from build123d import *

# Parameters (mm, degrees)
F1_DEPTH = 29
F2_R     = 10
F3_DEPTH = 20.001
F4_W     = 9.6138500422
F4_H     = 3
F5_DEPTH = 20.001
F7_D     = 6.3


with BuildPart() as f1:
    # F0 (on Top) → F1 (new body)
    with BuildSketch(Plane.XY):
        Polygon((20, 5), (15, 10), (-15, 10), (-20, 5), (-20, -5), (-15, -10), (15, -10), (20, -5), align=None)
    extrude(amount=F1_DEPTH)

    # F2 (on face) → F3 (cut, through all)
    with BuildSketch(Plane.XZ.offset(10)):
        with Locations((0, 13)):
            Circle(F2_R)
    extrude(amount=-F3_DEPTH, mode=Mode.SUBTRACT)

    # F4 (on face) → F5 (cut, through all)
    with BuildSketch(Plane.XZ.offset(10)):
        with Locations((-19.8069250211, 13)):
            Rectangle(F4_W, F4_H)
        with BuildLine():
            Line((-9.8868599666, 11.5), (-4.6138500422, 11.5))
            Line((-4.6138500422, 11.5), (-4.6138500422, 14.5))
            Line((-4.6138500422, 14.5), (-9.8868599666, 14.5))
            ThreePointArc((-9.8868599666, 14.5), (-10, 13), (-9.8868599666, 11.5))
        make_face()
        with BuildLine():
            Line((-15, 11.5), (-9.8868599666, 11.5))
            ThreePointArc((-9.8868599666, 11.5), (-10, 13), (-9.8868599666, 14.5))
            Line((-9.8868599666, 14.5), (-15, 14.5))
            Line((-15, 14.5), (-15, 11.5))
        make_face()
    extrude(amount=-F5_DEPTH, mode=Mode.SUBTRACT)

    # F7 (through all)
    with Locations(Plane.XY.offset(29)):
        with Locations((-15, 0), (15, 0)):
            Hole(F7_D / 2)


solid = f1.part
The listing builds one solid part. Answer for the finished solid, in the listing's coordinates (mm). A direction names the side the tool comes from. Round coordinates to 2 decimals unless told otherwise and drop trailing zeros. Write each loop counter-clockwise with the first axis right and the second up, starting at its lowest first coordinate (ties: lowest second). Pieces come first, ordered by that corner, then holes. Notation, with made-up numbers: (47.5, 10.25) - (62.5, 10.25) arc R35 cw to (62.5, 43.25) - close; hole circle Ø7 at (42, 5). An arc over 180 degrees is marked (long way). Use a Markdown table: item, result. Add a question column.
1. A flat-ended cylindrical pin translates along its axis: P1, Ø1, axis at x = 12.5, y = 4.5, coming from the -Z side. Find the tip coordinate at first contact, or state that the pin passes through.
2. The part is cut by section C-C (x = 0). Write down the section's boundary in (y, z).
3. The part is cut by section A-A (y = 0). Write down the section's boundary in (x, z).
4. A tool of negligible diameter and unlimited length cuts with its end or side. For faces 4 (the face through (-11.5, -0.1, 14.5)), 5 (the face through (-7, -10, 21)), from which of +Z, -Z, +X, -X, +Y, -Y can it reach the whole face along a straight path? Write none if from no direction.
5. Consider line 1 (Z direction, x = -17.5, y = -6.25); line 2 (Y direction, x = -15, z = 3.5); line 3 (X direction, y = 2.5, z = 20.5). Determine where each line is inside the solid, lowest interval first.
6. For a pull along Y with two mould halves and no side action, classify faces 1 (the face through (18.147, 0.138, 14.297)), 2 (the face through (-17, 8, 6)), 3 (the face through (-11.6, -0.1, 11.5)) as +Y half, -Y half, draft (parallel to the pull), parting line (faces both ways), or undercut.
7. The part is cut by section D-D (z = 17.25). Write down the section's boundary in (x, y), and give its area (3 significant figures).
8. The part is cut by section B-B (z = 13). Write down the section's boundary in (x, y), and give its area (3 significant figures).
Reported:
| question | item | result |
|---|---|---|
| 1 | P1 | z = 0 |
| 2 | outline | (-10, 0) - (10, 0) - (10, 3) - (-10, 3) - close; (-10, 23) - (10, 23) - (10, 29) - (-10, 29) - close |
| 3 | outline | (-20, 0) - (-18.15, 0) - (-18.15, 11.5) - (-20, 11.5) - close; (-20, 14.5) - (-18.15, 14.5) - (-18.15, 29) - (-20, 29) - close; (-11.85, 0) - (11.85, 0) - (11.85, 29) - (-11.85, 29) - (-11.85, 14.5) - (-9.89, 14.5) arc R10 cw (long way) to (-9.89, 11.5) - (-11.85, 11.5) - close; (18.15, 0) - (20, 0) - (20, 29) - (18.15, 29) - close |
| 4 | face 4 | -X, +Y, -Y |
| 4 | face 5 | +Z, -Z, +X, -X, -Y |
| 5 | line 1 | 0 to 11.5, 14.5 to 29 |
| 5 | line 2 | -10 to -3.15, 3.15 to 10 |
| 5 | line 3 | -20 to -16.92, -13.08 to -6.61, 6.61 to 13.08, 16.92 to 20 |
| 6 | face 1 | undercut |
| 6 | face 2 | +Y half |
| 6 | face 3 | draft |
| 7 | outline | (-20, -5) - (-15, -10) - (-9.05, -10) - (-9.05, 10) - (-15, 10) - (-20, 5) - close; (9.05, -10) - (15, -10) - (20, -5) - (20, 5) - (15, 10) - (9.05, 10) - close; hole circle Ø6.3 at (-15, 0); hole circle Ø6.3 at (15, 0) |
| 7 | area | 326 mm^2 |
| 8 | outline | (10, -10) - (15, -10) - (20, -5) - (20, 5) - (15, 10) - (10, 10) - close; hole circle Ø6.3 at (15, 0) |
| 8 | area | 144 mm^2 |
